Model file for the job. Use its own axes, mm. Round coordinates to 2 decimals unless told otherwise and drop trailing zeros. Use a Markdown table: item, result. Add a question column.
```python
from build123d import *

# Parameters (mm, degrees)
SKETCH1_W           = 50
SKETCH1_H           = 146
BOSS_EXTRUDE1_DEPTH = 6
SKETCH3_W           = 50
SKETCH3_H           = 146
SKETCH3_R           = 1.7
CUT_EXTRUDE1_DEPTH  = 78.395090284


with BuildPart() as part:
    # Sketch1 → Boss-Extrude1 (new body)
    with BuildSketch(Plane.XY):
        Rectangle(SKETCH1_W, SKETCH1_H)
    extrude(amount=BOSS_EXTRUDE1_DEPTH)

    # Sketch3 → Cut-Extrude1 (cut, through all)
    # profile 1 of 5: a face of its own
    with BuildSketch(Plane.XY.offset(6)):
        Rectangle(SKETCH3_W, SKETCH3_H)
        with BuildLine():
            Line((-18.157666585, 62.461107324), (-18.169843297, 52.461114738))
            Line((-18.169843297, 52.461114738), (2.830141135, 52.435543643))
            Line((2.830141135, 52.435543643), (2.780216616, 11.435574039))
            Line((2.780216616, 11.435574039), (-18.219767816, 11.461145134))
            Line((-18.219767816, 11.461145134), (-20.602879389, 2.095244868))
            add(Edge.make_bspline(
                [(-20.602879389, 2.095244868), (-20.020523896, 0.117608734), (-18.597491452, -3.334331588), (-16.904181184, -8.263198364), (-15.595665152, -12.546131745), (-14.456132729, -16.810408344), (-13.502980015, -20.975707084), (-12.475078727, -26.375577077), (-11.593046993, -32.660410116), (-10.802512336, -42.889860589), (-11.008756714, -54.642065179), (-12.153104447, -63.838427604), (-12.816272335, -67.795493305)],
                knots=[0, 0, 0, 0, 0.086646204, 0.157135059, 0.219373113, 0.275194629, 0.342966262, 0.399251523, 0.506628072, 0.609997758, 0.831095498, 1, 1, 1, 1], degree=3))
            ThreePointArc((-12.816272335, -67.795493305), (-9.012812454, -72.656301077), (-3.386129771, -70.119728338))
            add(Edge.make_bspline(
                [(-3.386129771, -70.119728338), (-2.21747594, -67.029455897), (-0.182430908, -61.43213239), (2.320638839, -54.010869169), (4.39612593, -47.471958806), (6.084233389, -41.826754396), (7.773371334, -35.827923865), (9.314485553, -30.006285299), (10.847177653, -23.777350088), (12.248531309, -17.633995633), (13.38184099, -12.246243723), (14.445923409, -6.813215488), (15.450948646, -1.273466268), (16.541323936, 5.397802811), (17.525796818, 12.227452617), (18.318292736, 18.577526245), (18.968243317, 24.556005739), (19.546819221, 30.747357743), (20.091144312, 37.979656821), (20.373774924, 43.153327808), (20.493418189, 45.880508448)],
                knots=[0, 0, 0, 0, 0.083335097, 0.150214343, 0.197536109, 0.256374009, 0.298827669, 0.354728647, 0.408266597, 0.460622921, 0.513659664, 0.547132194, 0.600265327, 0.655665944, 0.717630207, 0.774302923, 0.817071636, 0.86931356, 0.9311449, 1, 1, 1, 1], degree=3))
            ThreePointArc((20.493418189, 45.880508448), (20.406083271, 46.335184873), (20.123317244, 46.701792855))
            add(Edge.make_bspline(
                [(8.617522303, 71.930046937), (8.590710324, 70.931587333), (8.616247935, 68.508726225), (8.97509159, 65.334163001), (9.675355593, 62.166917416), (10.407826162, 59.878461992), (11.375637803, 57.567082564), (12.476705695, 55.420888781), (13.985734658, 53.073760845), (15.699091005, 50.90924769), (17.727100256, 48.757794454), (19.223608489, 47.429602703), (20.123317244, 46.701792855)],
                knots=[0, 0, 0, 0, 0.10400348, 0.252210124, 0.331596335, 0.441573044, 0.501852928, 0.592428261, 0.692389888, 0.791956146, 0.879471991, 1, 1, 1, 1], degree=3))
            ThreePointArc((8.617522303, 71.930046937), (8.006083211, 72.878510262), (6.900295351, 72.653402178))
            add(Edge.make_bspline(
                [(-18.157666585, 62.461107324), (-16.595787428, 62.40054525), (-13.772759201, 62.464261258), (-9.697592278, 63.074582136), (-6.3235109, 64.014176015), (-3.330757616, 65.219156255), (-0.94481153, 66.454321846), (1.113119903, 67.745229422), (3.761030335, 69.658518488), (5.631814544, 71.346079367), (6.900295351, 72.653402178)],
                knots=[0, 0, 0, 0, 0.167942372, 0.302841242, 0.441808799, 0.543310726, 0.649111052, 0.730099181, 0.804199887, 1, 1, 1, 1], degree=3))
        make_face(mode=Mode.SUBTRACT)
    # profile 2 of 5: a face of its own
    with BuildSketch(Plane.XY.offset(6)):
        with Locations((-12.724033742, 7.954450537)):
            Circle(SKETCH3_R)
    # profile 3 of 5: a face of its own
    with BuildSketch(Plane.XY.offset(6)):
        with Locations((-2.724041156, 7.942273825)):
            Circle(SKETCH3_R)
    # profile 4 of 5: a face of its own
    with BuildSketch(Plane.XY.offset(6)):
        with Locations((-12.665585525, 55.954414952)):
            Circle(SKETCH3_R)
    # profile 5 of 5: a face of its own
    with BuildSketch(Plane.XY.offset(6)):
        with Locations((-2.665592939, 55.94223824)):
            Circle(SKETCH3_R)
    extrude(amount=-CUT_EXTRUDE1_DEPTH, mode=Mode.SUBTRACT)


solid = part.part
```
1) Wall check: probe 1 along X at (y, z) = (56.5, 3.25); probe 2 along Y at (x, z) = (-4, 2); probe 3 along Y at (x, z) = (-7, 2). Give the ranges that are in metal, low to high. Write a range as from..to.
2) Pull direction X, two halves, no side cores. Call faces 1 (the face through (0, 1, 0)), 2 (the face through (-9.103, -72.633, 3.042)), 3 (the face through (-11.881, 54.446, 3.042)), 4 (the face through (-1.154, 7.291, 3.042)): +X half, -X half, draft (parallel to the pull), parting line (faces both ways), or undercut.
3) Pin check, flat tips, straight feed: pin 1 Ø4.5 at (x, y) = (-2.72, 7.94) entering from +Z; pin 2 Ø2.5 at (x, y) = (-2.67, 55.94) entering from -Z; pin 3 Ø1.5 at (y, z) = (-12.5, 4.5) entering from +X. Stop position of each tip, or through.
4) Cut at A-A on z = 1.25. Count the separate pieces of the cut face and the enclosed holes in it, and give its area (3 significant figures).
Established:
| question | item | result |
|---|---|---|
| 1 | probe 1 | x = -18.16..-14.28, -11.06..-4.27, -1.06..11.94 |
| 1 | probe 2 | y = -71.03..6.82, 9.07..11.44, 52.44..54.89, 57..64.97 |
| 1 | probe 3 | y = -72.73..11.45, 52.45..63.86 |
| 2 | face 1 | draft |
| 2 | face 2 | parting line |
| 2 | face 3 | undercut |
| 2 | face 4 | undercut |
| 3 | pin 1 | stops at z = 6 |
| 3 | pin 2 | passes through |
| 3 | pin 3 | stops at x = 13.47 |
| 4 | separate pieces | 1 |
| 4 | enclosed holes | 4 |
| 4 | area | 2,880 mm^2 |
